CAD build for the part. Positions are in the model's coordinates, mm. Give positions to 0.01 mm unless a question says otherwise; leave off trailing zeros. Write each loop counter-clockwise with the first axis right and the second up, starting at its lowest first coordinate (ties: lowest second). Pieces come first, ordered by that corner, then holes. Notation, with made-up numbers: (-23.5, -5.75) - (-9.5, -5.75) arc R26 ccw to (-9.5, 31.25) - close; hole circle Ø10 at (16, 1.25). An arc over 180 degrees is marked (long way). Put each result on its own line as item: value. Start each with the question number.
1. Cut at B-B on y = -5. Give the number of separate pieces and of enclosed holes in the cut face, and give its area (3 significant figures).
2. Cut at C-C on x = 0. List the corners of the cut face in (y, z) (3 decimals), and give its area (3 significant figures).
3. Wall check: line 1 (Z direction, x = 107.95, y = -2.5) (3 decimals); line 2 (Z direction, x = 114, y = -0.5) (3 decimals). Give the ranges that are in metal, low to high.
from build123d import *

# Parameters (mm, degrees)
F0_W     = 431.8
F0_H     = 82.55
F1_DEPTH = 6.35
F3_DEPTH = 6.35
F5_DEPTH = 6.35


with BuildPart() as f1:
    # F0 (on Front) → F1 (new body)
    with BuildSketch(Plane.XZ):
        Rectangle(F0_W, F0_H)
    extrude(amount=F1_DEPTH)

    # F2 (on face) → F3 (cut, through all)
    with BuildSketch(Plane.XZ.offset(6.35)):
        with BuildLine():
            ThreePointArc((-93.6625, 0), (-107.95, 14.2875), (-122.2375, 0))
            Line((-122.2375, 0), (-93.6625, 0))
        make_face()
        with BuildLine():
            ThreePointArc((117.475, 0), (107.95, 9.525), (98.425, 0))
            Line((98.425, 0), (117.475, 0))
        make_face()
        with BuildLine():
            Line((117.475, 0), (98.425, 0))
            ThreePointArc((98.425, 0), (107.95, -9.525), (117.475, 0))
        make_face()
        with BuildLine():
            ThreePointArc((9.525, 0), (0, 9.525), (-9.525, 0))
            Line((-9.525, 0), (9.525, 0))
        make_face()
        with BuildLine():
            Line((9.525, 0), (-9.525, 0))
            ThreePointArc((-9.525, 0), (0, -9.525), (9.525, 0))
        make_face()
        with BuildLine():
            Line((-93.6625, 0), (-122.2375, 0))
            ThreePointArc((-122.2375, 0), (-107.95, -14.2875), (-93.6625, 0))
        make_face()
    extrude(amount=-F3_DEPTH, mode=Mode.SUBTRACT)

    # F4 (on face) → F5 (cut, through all)
    with BuildSketch(Plane.XZ.offset(6.35)):
        with BuildLine():
            Line((-123.10745, -15.15745), (-123.10745, -13.13815))
            ThreePointArc((-123.10745, -13.13815), (-124.535311, -16.585311), (-121.08815, -15.15745))
            Line((-121.08815, -15.15745), (-123.10745, -15.15745))
        make_face()
        with BuildLine():
            ThreePointArc((-121.08815, -15.15745), (-121.679589, -13.729589), (-123.10745, -13.13815))
            Line((-123.10745, -13.13815), (-123.10745, -15.15745))
            Line((-123.10745, -15.15745), (-121.08815, -15.15745))
        make_face()
        with BuildLine():
            ThreePointArc((-90.77325, -15.15745), (-91.364689, -13.729589), (-92.79255, -13.13815))
            Line((-92.79255, -13.13815), (-92.79255, -15.15745))
            Line((-92.79255, -15.15745), (-94.81185, -15.15745))
            ThreePointArc((-94.81185, -15.15745), (-92.79255, -17.17675), (-90.77325, -15.15745))
        make_face()
        with BuildLine():
            Line((-92.79255, -15.15745), (-92.79255, -13.13815))
            ThreePointArc((-92.79255, -13.13815), (-94.220411, -13.729589), (-94.81185, -15.15745))
            Line((-94.81185, -15.15745), (-92.79255, -15.15745))
        make_face()
        with BuildLine():
            Line((-92.79255, 15.15745), (-94.81185, 15.15745))
            ThreePointArc((-94.81185, 15.15745), (-94.220411, 13.729589), (-92.79255, 13.13815))
            Line((-92.79255, 13.13815), (-92.79255, 15.15745))
        make_face()
        with BuildLine():
            ThreePointArc((-90.77325, 15.15745), (-92.79255, 17.17675), (-94.81185, 15.15745))
            Line((-94.81185, 15.15745), (-92.79255, 15.15745))
            Line((-92.79255, 15.15745), (-92.79255, 13.13815))
            ThreePointArc((-92.79255, 13.13815), (-91.364689, 13.729589), (-90.77325, 15.15745))
        make_face()
        with BuildLine():
            ThreePointArc((-123.10745, 13.13815), (-121.679589, 13.729589), (-121.08815, 15.15745))
            Line((-121.08815, 15.15745), (-123.10745, 15.15745))
            Line((-123.10745, 15.15745), (-123.10745, 13.13815))
        make_face()
        with BuildLine():
            Line((-123.10745, 15.15745), (-121.08815, 15.15745))
            ThreePointArc((-121.08815, 15.15745), (-124.535311, 16.585311), (-123.10745, 13.13815))
            Line((-123.10745, 13.13815), (-123.10745, 15.15745))
        make_face()
    extrude(amount=-F5_DEPTH, mode=Mode.SUBTRACT)


solid = f1.part
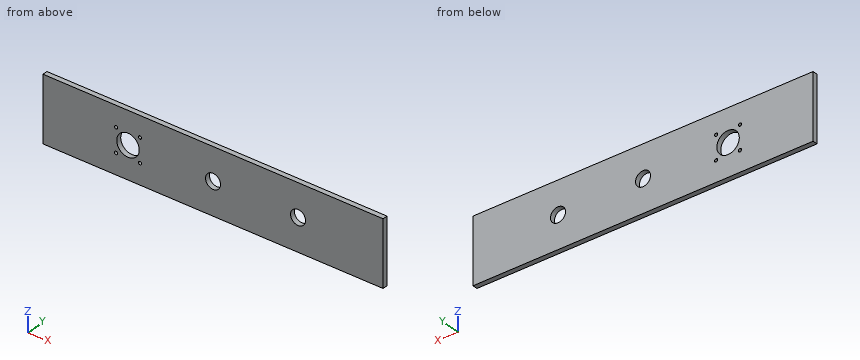
Report:
1. separate pieces: 1
1. enclosed holes: 7
1. area: 34,400 mm²
2. outline: (-6.35, -41.275) - (0, -41.275) - (0, -9.525) - (-6.35, -9.525) - close; (-6.35, 9.525) - (0, 9.525) - (0, 41.275) - (-6.35, 41.275) - close
2. area: 403 mm²
3. line 1: z = -41.275 to -9.525, 9.525 to 41.275
3. line 2: z = -41.275 to -7.357, 7.357 to 41.275
